```python
from build123d import *

# Parameters (mm, degrees)
F0_W          = 127
F0_H          = 30.127738
F1_DEPTH      = 25.4
F1_DEPTH_BACK = 25.4
F2_R          = 19.05
F3_DEPTH      = 15.064869
F3_DEPTH_BACK = 15.063869
F4_R          = 5.08


with BuildPart() as f1:
    # F0 (on Front) → F1 (new body, two sides)
    with BuildSketch(Plane.XZ) as f1_sk:
        Rectangle(F0_W, F0_H)
        Polygon((-63.5, -15.063869), (-63.5, 15.063869), (-125.187356, 0), align=None)
    extrude(amount=F1_DEPTH)
    extrude(f1_sk.sketch, amount=-F1_DEPTH_BACK)

    # F2 (on Top) → F3 (cut, two sides)
    with BuildSketch(Plane.XY) as f3_sk:
        Circle(F2_R)
    extrude(amount=F3_DEPTH, mode=Mode.SUBTRACT)
    extrude(f3_sk.sketch, amount=-F3_DEPTH_BACK, mode=Mode.SUBTRACT)

    # F4
    f4_edges = [f1.edges().sort_by_distance(p)[0] for p in [
        (-125.187356, 0, 0),
    ]]
    fillet(f4_edges, radius=F4_R)


solid = f1.part
```
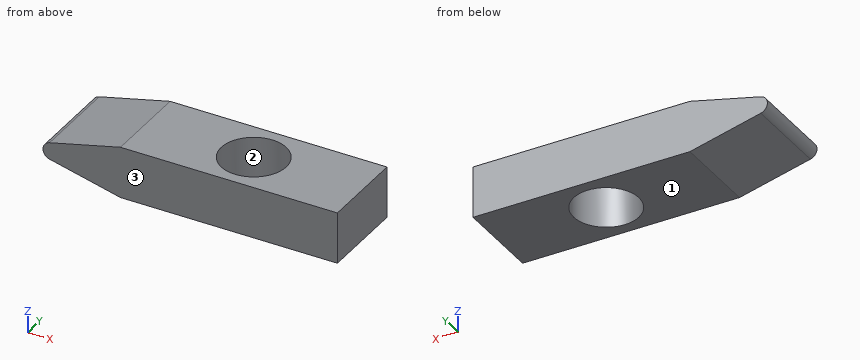
The model under review builds one solid part; all positions refer to its coordinate system, in mm. Face numbers are marked on the shaded views. Round coordinates to 2 decimals unless told otherwise and drop trailing zeros. Loops run counter-clockwise (first coordinate to the right, second up) from the corner with the lowest first, then second, coordinate; pieces in that order, holes last.
Item 1: Take a section at C-C (z = 2.5). Write out the cut boundary in (x, y).
Determined:
outline: (-108.2, -25.4) - (63.5, -25.4) - (63.5, 25.4) - (-108.2, 25.4) - close; hole circle Ø38.1 at (0, 0)
Item 2: Clearance check with flat-ended pins moving along their axes: pin 1 Ø10 at (y, z) = (6, 7.5) entering from -X; pin 2 Ø1 at (x, y) = (-87.5, 0.5) entering from +Z; pin 3 Ø3 at (x, y) = (-91, -13) entering from +Z. State where each tip first meets the part, or that it passes through.
Determined:
pin 1: stops at x = -108.2
pin 2: stops at z = 9.33
pin 3: stops at z = 8.71
Item 3: Take a section at D-D (y = 22.5). Write out the cut boundary in (x, z).
Determined:
outline: (-104.98, -4.93) - (-63.5, -15.06) - (63.5, -15.06) - (63.5, 15.06) - (-63.5, 15.06) - (-104.98, 4.93) arc R5.08 ccw to start
Item 4: For line 1 (Y direction, x = 0, z = 2); line 2 (X direction, y = -12, z = -3.5); line 3 (X direction, y = 0, z = -2), list the stretches that pass through material, from the lowest coordinate up.
Determined:
line 1: y = -25.4 to -19.05, 19.05 to 25.4
line 2: x = -107.46 to -14.8, 14.8 to 63.5
line 3: x = -108.44 to -19.05, 19.05 to 63.5
Item 5: Take a section at A-A (y = 0). Write out the cut boundary in (x, z), then the cut area to 3 significant figures.
Determined:
outline: (-104.98, -4.93) - (-63.5, -15.06) - (-19.05, -15.06) - (-19.05, 15.06) - (-63.5, 15.06) - (-104.98, 4.93) arc R5.08 ccw to start; (19.05, -15.06) - (63.5, -15.06) - (63.5, 15.06) - (19.05, 15.06) - close
area: 3,540 mm2
Item 6: Mouldability with a two-part tool opening along Y and no side actions: class the marked faces 1, 2 and 3 as released by +Y, released by -Y, zero draft, split by the parting line, or undercut.
Determined:
face 1: zero draft
face 2: undercut
face 3: released by -Y
Item 7: Take a section at B-B (x = -9). Write out the cut boundary in (y, z), then the cut area to 3 significant figures.
Determined:
outline: (-25.4, -15.06) - (-16.79, -15.06) - (-16.79, 15.06) - (-25.4, 15.06) - close; (16.79, -15.06) - (25.4, -15.06) - (25.4, 15.06) - (16.79, 15.06) - close
area: 519 mm2
